The figure shows three views and two pictorial views of one solid part (mm, origin at its lowest corner). Answer the questions. A direction names the side the tool comes from. Give positions to 0.01 mm unless a question says otherwise; leave off trailing zeros. Loops run counter-clockwise (first coordinate to the right, second up) from the corner with the lowest first, then second, coordinate; pieces in that order, holes last. Notation, with made-up numbers: M 8.25,-19 L 57.25,-19 A12 ccw 57.25,-12 Z; hole C 76,-33 d8. An arc over 180 degrees is marked long. One line per item, written item: value. Start each with the question number.
Q1. Consider L1, parallel to Z at x = 12.25, y = 0.25; L2, parallel to X at y = 0.65, z = 12.5; L3, parallel to Z at x = 17.5, y = 1.4. Determine where each line is inside the solid, lowest interval first.
Q2. The mould has two halves that part along Z. Classify the marked faces 1, 2 and 3: +Z half, -Z half, draft (parallel to the pull), parting line (faces both ways), or undercut.
Q3. A cutting plane is placed at A-A, the plane x = 12.5. Determine the outline of the cut face in (y, z).
Q4. Flat-ended cylindrical pins translate along their axes: pin 1 (1 mm diameter, centred on y = 1.5, z = 6.5, fed in from -X) (3 decimals); pin 2 (0.6 mm diameter, centred on x = 18.5, y = 1, fed in from -Z) (1 decimal); pin 3 (0.6 mm diameter, centred on x = 18.5, y = 0.5, fed in from +Z) (1 decimal); pin 4 (12 mm diameter, centred on x = 9.5, z = 15, fed in from -Y). Find the tip coordinate at first contact, or state that the pin passes through.
Q5. A cutting plane is placed at B-B, the plane y = 0.9. Determine the outline of the cut face in (x, z) (3 decimals), and give its area (3 significant figures).
Q6. For the marked faces 4 and 5, determine the directions among +Z, -Z, +X, -X, +Y, -Y from which every point of the face is accessible in a straight line to the end or side of a thin tool.
Q7. A cutting plane is placed at C-C, the plane x = 18.75. Determine the outline of the cut face in (y, z), and give its area (3 significant figures).
Q8. A cutting plane is placed at D-D, the plane z = 12.5. Determine the outline of the cut face in (x, y), and give its area (3 significant figures).
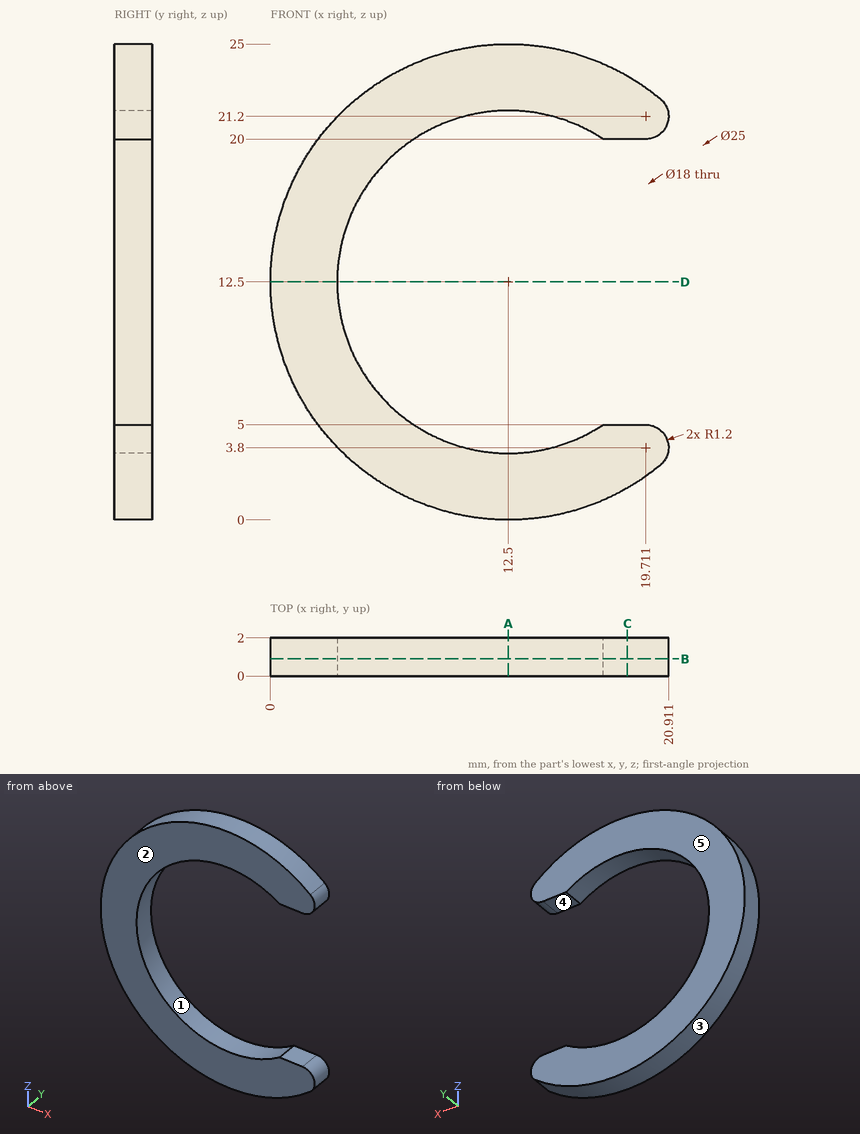
Answer block:
1. L1: 0 to 3.5, 21.5 to 25
1. L2: 0 to 3.5
1. L3: 1.04 to 5, 20 to 23.96
2. face 1: undercut
2. face 2: draft
2. face 3: parting line
3. outline: M 0,0 L 2,0 L 2,3.5 L 0,3.5 Z; M 0,21.5 L 2,21.5 L 2,25 L 0,25 Z
4. pin 1: x = 1.275
4. pin 2: z = 1.4
4. pin 3: z = 23.6
4. pin 4: y = 0
5. outline: M 17.475,5 A9 cw long 17.475,20 L 19.711,20 A1.2 ccw 20.477,22.124 A12.5 ccw long 20.477,2.876 A1.2 ccw 19.711,5 Z
5. area: 174 mm^2
6. face 4: +X, +Y, -Y
6. face 5: +Z, -Z, +X, -X, +Y
7. outline: M 0,1.67 L 2,1.67 L 2,5 L 0,5 Z; M 0,20 L 2,20 L 2,23.33 L 0,23.33 Z
7. area: 13.3 mm^2
8. outline: M 0,0 L 3.5,0 L 3.5,2 L 0,2 Z
8. area: 7.00 mm^2
